Design review of the part built by this model. Coordinates are the model's own, in mm. Coordinates: 2 decimals unless noted, no trailing zeros. Loops run counter-clockwise (first coordinate to the right, second up) from the corner with the lowest first, then second, coordinate; pieces in that order, holes last. Notation, with made-up numbers: M -23,66.5 L -17,66.5 A24 ccw -17,86.5 Z; hole C 82,-37.75 d5. An arc over 180 degrees is marked long. Answer as a JSON object with one key per item and string values. Group by question number.
1. Consider section D-D (x = 97). State the section outline as (y, z) points, then the cut area to 3 significant figures.
2. Consider section A-A (y = 60). State the section outline as (x, z) points, then the cut area to 3 significant figures.
3. To check wall thickness, follow probe 1 along Y at (x, z) = (6, 0); probe 2 along Y at (x, z) = (21, -48.5). State the ranges of each line that lie inside material, in increasing order.
4. Consider section C-C (y = 130). State the section outline as (x, z) points, then the cut area to 3 significant figures.
5. Consider section B-B (z = 0). State the section outline as (x, y) points, then the cut area to 3 significant figures.
6. Insertion check: pin 1 (4 mm diameter, centred on y = 36.5, z = 25, fed in from +X); pin 2 (11 mm diameter, centred on y = 2.5, z = 18, fed in from +X); pin 3 (13.5 mm diameter, centred on y = 60, z = 0, fed in from +X); pin 4 (12 mm diameter, centred on x = 37.5, z = 22, fed in from +Y). Each pin has a flat end and moves straight along its axis. Give the tip position at first contact, or say it passes through.
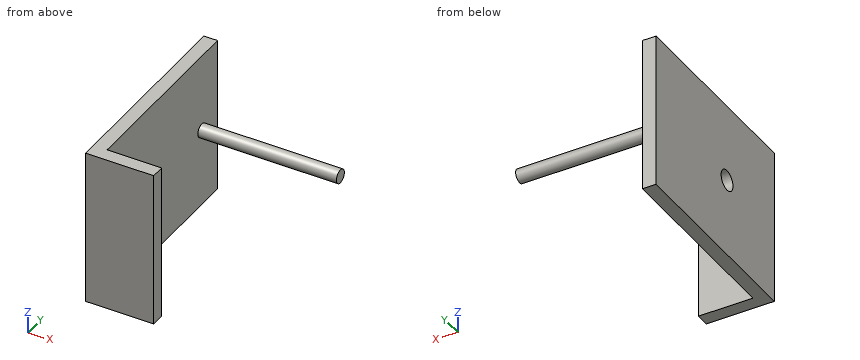
from build123d import *

# Parameters (mm, degrees)
BOSS_EXTRUDE1_DEPTH = 57.5
SKETCH2_R           = 7.5
CUT_EXTRUDE1_DEPTH  = 51
SKETCH3_R           = 5
BOSS_EXTRUDE2_DEPTH = 101.780663763


with BuildPart() as part:
    # Sketch1 → Boss-Extrude1 (new body, symmetric)
    with BuildSketch(Plane.XY):
        Polygon((0, 150), (0, 0), (50, 0), (50, 10), (10, 10), (10, 150), align=None)
    extrude(amount=BOSS_EXTRUDE1_DEPTH, both=True)

    # Sketch2 → Cut-Extrude1 (cut, through all)
    with BuildSketch(Plane.ZY):
        with Locations((0, 60)):
            Circle(SKETCH2_R)
    extrude(amount=-CUT_EXTRUDE1_DEPTH, mode=Mode.SUBTRACT)

    # Sketch3 → Boss-Extrude2 (add)
    with BuildSketch(Plane(origin=(10, 0, 0), x_dir=(0, 0, -1), z_dir=(1, 0, 0))):
        with Locations((0, 130)):
            Circle(SKETCH3_R)
    extrude(amount=BOSS_EXTRUDE2_DEPTH)


solid = part.part
Findings below:
{
 "1": {"outline": "C 130,0 d10", "area": "78.5 mm^2"},
 "2": {"outline": "M 0,-57.5 L 10,-57.5 L 10,-7.5 L 0,-7.5 Z; M 0,7.5 L 10,7.5 L 10,57.5 L 0,57.5 Z", "area": "1,000 mm^2"},
 "3": {"probe 1": "y = 0 to 52.5, 67.5 to 150", "probe 2": "y = 0 to 10"},
 "4": {"outline": "M 0,-57.5 L 10,-57.5 L 10,-5 L 111.78,-5 L 111.78,5 L 10,5 L 10,57.5 L 0,57.5 Z", "area": "2,170 mm^2"},
 "5": {"outline": "M 0,0 L 50,0 L 50,10 L 10,10 L 10,52.5 L 0,52.5 Z; M 0,67.5 L 10,67.5 L 10,125 L 111.78,125 L 111.78,135 L 10,135 L 10,150 L 0,150 Z", "area": "2,770 mm^2"},
 "6": {"pin 1": "stops at x = 10", "pin 2": "stops at x = 50", "pin 3": "passes through", "pin 4": "stops at y = 10"}
}
